Autodesk Inventor part; units mm, degrees
ref_plane "YZ Plane" through (0, 0, 0) normal (1, 0, 0) x (0, 1, 0)
ref_plane "XZ Plane" through (0, 0, 0) normal (0, 1, 0) x (-1, 0, 0)
ref_plane "XY Plane" through (0, 0, 0) normal (0, 0, 1) x (1, 0, 0)
sketch "Szkic3" plane through (0, 0, 0) normal (0, 1, 0) x (-1, 0, 0)
  circle A0 centre (0, 0) radius 27.25
  dimension "d7" = 54.5
extrude "Wyciągnięcie proste3" add sketch "Szkic3" along normal blind 2
sketch "Szkic4" plane through (0, 2, 0) normal (0, 1, 0) x (1, 0, 0)
  circle A0 centre (-22.5, 0) radius 3.4
  point P0 (0, 0)
  dimension "d10" = 22.5
  dimension "d16" = 6.8
extrude "Wyciągnięcie proste4" add sketch "Szkic4" along normal blind 5
pattern_circular "Szyk kołowy1" count 10 over 360 about axis through (0, 0, 0) along (0, 1, 0) of "Wyciągnięcie proste4"
sketch "Szkic5" plane through (0, 0, 0) normal (0, -1, 0) x (1, 0, 0)
  circle A0 centre (22.5, 0) radius 1.45
  point P0 (0, 0)
  dimension "d17" = 2.9
extrude "Wyciągnięcie proste5" cut sketch "Szkic5" against normal up to surface (7 mm away)
pattern_circular "Szyk kołowy2" count 5 over 360 about axis through (0, 0, 0) along (0, 1, 0) of "Wyciągnięcie proste5"
sketch "Szkic6" plane through (0, 2, 0) normal (0, 1, 0) x (1, 0, 0)
  circle A0 centre (0, 0) radius 16.25
  dimension "d23" = 32.5
extrude "Wyciągnięcie proste6" cut sketch "Szkic6" against normal up to surface (2 mm away)
properties part number "OutputShaft1_3DPrint"
Verification items for the finished model (mm, model axes). A direction names the side the tool comes from. Round coordinates to 2 decimals unless told otherwise and drop trailing zeros. Order: outer loops, then holes, each group sorted by start corner. A loop starts at its lowest first (then second) coordinate and runs counter-clockwise, first axis right, second up.
1. Section check D-D on z = 7.5. Record the cut outline in (x, y).
Final values:
outline: (-26.2, 0) - (-14.42, 0) - (-14.42, 2) - (-26.2, 2) - close; (14.42, 0) - (26.2, 0) - (26.2, 2) - (14.42, 2) - close
2. Release check for a two-part mould opening along Z. For faces 3 (the cylindrical face through (21.58, 4.46, 12.84)), 4 (the flat face through (18, 7, 13)) record: +Z half, -Z half, draft (parallel to the pull), parting line (faces both ways), or undercut.
Final values:
face 3: undercut
face 4: draft
3. Thickness scan on L1, parallel to X at y = 4.5, z = -21.5; L2, parallel to Z at x = 7, y = 2.25; L3, parallel to Z at x = 0, y = 0.9. Record the ranges inside material, lowest first.
Final values:
L1: x = -10.35 to -3.55, 3.55 to 5.51, 8.4 to 10.35
L2: z = -24.8 to -22.85, -19.95 to -18, 18 to 19.95, 22.85 to 24.8
L3: z = -27.25 to -16.25, 16.25 to 27.25
4. Section check A-A on z = 0. Record the cut outline in (x, y), then the cut area to 3 significant figures.
Final values:
outline: (-27.25, 0) - (-16.25, 0) - (-16.25, 2) - (-19.1, 2) - (-19.1, 7) - (-25.9, 7) - (-25.9, 2) - (-27.25, 2) - close; (16.25, 0) - (21.05, 0) - (21.05, 7) - (19.1, 7) - (19.1, 2) - (16.25, 2) - close; (23.95, 0) - (27.25, 0) - (27.25, 2) - (25.9, 2) - (25.9, 7) - (23.95, 7) - close
area: 91.7 mm2
5. Access from +Z, -Z, +X, -X, +Y, -Y to the whole of each face (thin tool, end or side, straight path). Record for faces 1 (the cylindrical face through (19.36, 4.46, 1.3)), 2 (the flat face through (6, 7, -20)).
Final values:
face 1: +Y
face 2: +Z, -Z, +X, -X, +Y
6. Section check B-B on x = 0. Record the cut outline in (y, z), then the cut area to 3 significant figures.
Final values:
outline: (0, -27.25) - (2, -27.25) - (2, -16.25) - (0, -16.25) - close; (0, 16.25) - (2, 16.25) - (2, 27.25) - (0, 27.25) - close
area: 44.0 mm2
7. Go/stop test with flat-tipped pins: P1, Ø3, axis at x = 11, z = 20.5, coming from the +Y side; P2, Ø3, axis at x = 17.5, z = 21.5, coming from the +Y side; P3, Ø1.5, axis at y = 4.5, z = -10, coming from the +X side; P4, Ø3, axis at x = -2.5, y = 6, coming from the -Z side. Record where each tip stops, or that it passes through.
Final values:
P1: stops at y = 7
P2: stops at y = 2
P3: stops at x = 20.53
P4: stops at z = -23.08
